from build123d import *

# Parameters (mm, degrees)
SKETCH1_R           = 12.5
BOSS_EXTRUDE4_DEPTH = 625.3
SKETCH4_R           = 5
CUT_EXTRUDE2_DEPTH  = 312.65
SKETCH5_R           = 17.5
SKETCH5_R_2         = 12.5
BOSS_EXTRUDE6_DEPTH = 17.5
SKETCH7_R           = 12.5
CUT_EXTRUDE4_DEPTH  = 17.5


with BuildPart() as part:
    # Sketch1 → Boss-Extrude4 (new body)
    with BuildSketch(Plane.XY):
        Circle(SKETCH1_R)
    extrude(amount=BOSS_EXTRUDE4_DEPTH)

    # Sketch4 → Cut-Extrude2 (cut, symmetric)
    with BuildSketch(Plane(origin=(0, 0, 0), x_dir=(0, 0, -1), z_dir=(1, 0, 0))):
        with Locations((-312.65, 0)):
            Circle(SKETCH4_R)
    extrude(amount=CUT_EXTRUDE2_DEPTH, both=True, mode=Mode.SUBTRACT)

    # Sketch5 → Boss-Extrude6 (add, symmetric)
    with BuildSketch(Plane(origin=(0, 0, 0), x_dir=(0, 0, -1), z_dir=(1, 0, 0))):
        Circle(SKETCH5_R)
        Circle(SKETCH5_R_2, mode=Mode.SUBTRACT)
        with Locations((-625.3, 0)):
            Circle(SKETCH5_R)
        with Locations((-625.3, 0)):
            Circle(SKETCH5_R_2, mode=Mode.SUBTRACT)
    extrude(amount=BOSS_EXTRUDE6_DEPTH, both=True)

    # Sketch7 → Cut-Extrude4 (cut, symmetric)
    with BuildSketch(Plane(origin=(0, 0, 0), x_dir=(0, 0, -1), z_dir=(1, 0, 0))):
        Circle(SKETCH7_R)
        with Locations((-625.3, 0)):
            Circle(SKETCH7_R)
    extrude(amount=CUT_EXTRUDE4_DEPTH, both=True, mode=Mode.SUBTRACT)


solid = part.part
Source: CAD feature listing. Evaluate the final solid. Frame: model axes, mm. A direction names the side the tool comes from. Coordinates: 2 decimals unless noted, no trailing zeros. Order: outer loops, then holes, each group sorted by start corner. A loop starts at its lowest first (then second) coordinate and runs counter-clockwise, first axis right, second up.
Item 1: Cut plane B-B (x = 0). Return loops of the section in (y, z), plus the area to 3 significant figures.
Output values:
outline: (-12.5, 12.25) arc R17.5 ccw (long way) to (12.5, 12.25) - (12.5, 613.05) arc R17.5 ccw (long way) to (-12.5, 613.05) - close; hole circle Ø25 at (0, 0); hole circle Ø25 at (0, 625.3); hole circle Ø10 at (0, 312.65)
area: 15,700 mm2
Item 2: Set-up query: faces 1 (the face through (-17.5, -11, -8)), 2 (the face through (11.923, 3.755, 308.444)). Return all of +Z, -Z, +X, -X, +Y, -Y with unobstructed straight access to the full face (end or side cutting, diameter ignored); none if empty.
Output values:
face 1: +Z, -Z, -X, +Y, -Y
face 2: none
Item 3: Pull-direction query (Z, two-part tool) for faces 3 (the face through (-0.245, -4.788, 613.753)), 4 (the face through (17.5, -8, 614)); classes: pulls with the +Z half, pulls with the -Z half, needs draft (parallel to the pull), parting line crosses it, or undercut.
Output values:
face 3: undercut
face 4: needs draft
Item 4: Cut plane A-A (z = 0). Return loops of the section in (x, y).
Output values:
outline: (-17.5, -17.5) - (17.5, -17.5) - (17.5, -12.5) - (-17.5, -12.5) - close; (-17.5, 12.5) - (17.5, 12.5) - (17.5, 17.5) - (-17.5, 17.5) - close
Item 5: Material intervals for line 1 (Z direction, x = 5.5, y = 4); line 2 (Y direction, x = 8, z = 0); line 3 (Y direction, x = 11.5, z = 319), sorted ascending.
Output values:
line 1: z = -17.04 to -11.84, 11.84 to 309.65, 315.65 to 613.46, 637.14 to 642.34
line 2: y = -17.5 to -12.5, 12.5 to 17.5
line 3: y = -4.9 to 4.9
Item 6: First-contact query: P1, Ø10, axis at x = 7.5, z = 241.5, coming from the +Y side; P2, Ø4, axis at y = -3, z = 254.5, coming from the +X side; P3, Ø12, axis at y = -9, z = 76.5, coming from the -X side. Flat tips, straight axial feed; report the tip coordinate or a pass-through.
Output values:
P1: stops at y = 12.25
P2: stops at x = 12.46
P3: stops at x = -12.13
Item 7: Cut plane C-C (z = 174.5). Return loops of the section in (x, y), plus the area to 3 significant figures.
Output values:
outline: circle Ø25 at (0, 0)
area: 491 mm2
